CAD build for the part. Positions are in the model's coordinates, mm. Face numbers are marked on the shaded views. A direction names the side the tool comes from. Round coordinates to 2 decimals unless told otherwise and drop trailing zeros. Loops run counter-clockwise (first coordinate to the right, second up) from the corner with the lowest first, then second, coordinate; pieces in that order, holes last.
```python
from build123d import *

# Parameters (mm, degrees)
F3_D = 12
F4_R = 2
F5_R = 4


with BuildPart() as f1:
    # F0 (on Front) → F1 (revolve)
    with BuildSketch(Plane.XZ):
        Polygon((22, 17), (17.25, 17), (17.25, 0), (47.5, 0), (47.5, 10), (22, 10), align=None)
    revolve(axis=Axis((0, 0, 4.398516), (0, 0, -1)))

    # F3 (through all)
    with Locations(Plane.XY.offset(10)):
        with Locations((-26.516504, 26.516504), (-26.516504, -26.516504), (26.516504, -26.516504), (26.516504, 26.516504)):
            Hole(F3_D / 2)

    # F4
    f4_edges = [f1.edges().sort_by_distance(p)[0] for p in [
        (-22, 0, 17),
        (-47.5, 0, 10),
    ]]
    fillet(f4_edges, radius=F4_R)

    # F5
    f5_edges = [f1.edges().sort_by_distance(p)[0] for p in [
        (-22, 0, 10),
    ]]
    fillet(f5_edges, radius=F5_R)


solid = f1.part
```
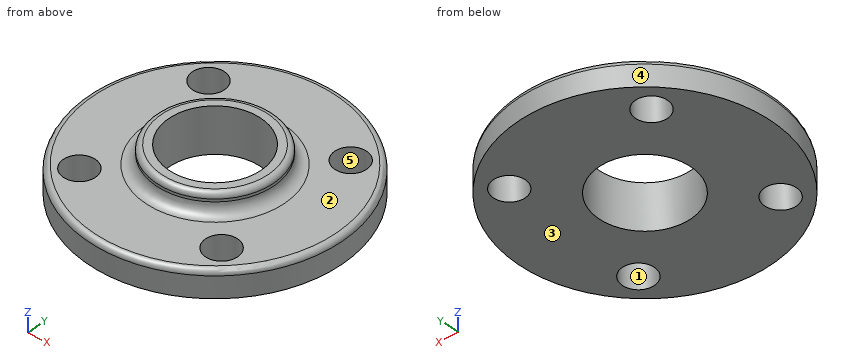
Item 1: Flat gauge pins, fed straight in: P1, Ø11, axis at x = -26.52, y = -26.52, coming from the -Z side; P2, Ø3, axis at x = -21.5, z = 7, coming from the -Y side; P3, Ø5, axis at x = 19.5, z = 6.5, coming from the -Y side; P4, Ø2, axis at x = 21, y = 5, coming from the +Z side. Where does each tip first touch, or does it go through?
Answers follow:
P1: passes through
P2: stops at y = -43.08
P3: stops at y = -44.35
P4: stops at z = 16.91
Item 2: Cut at D-D, the plane x = 31. State how many separate pieces and enclosed holes the cut face has, plus the area to 3 significant figures.
Answers follow:
separate pieces: 3
enclosed holes: 0
area: 558 mm2
Item 3: 3-axis set-ups, long thin cutter, end or side, ignore diameter. For the marked faces 1 and 2: which of +Z, -Z, +X, -X, +Y, -Y reach the whole face in a straight line?
Answers follow:
face 1: +Z, -Z
face 2: +Z
Item 4: Two-plate mould, pull along Y, no slides. Class the marked faces 3, 4 and 5: released by +Y, released by -Y, zero draft, split by the parting line, or undercut.
Answers follow:
face 3: zero draft
face 4: split by the parting line
face 5: undercut
Item 5: Cut at C-C, the plane z = 2.5. Give the cut face in (x, y), plus the area to 3 significant figures.
Answers follow:
outline: circle Ø95 at (0, 0); hole circle Ø12 at (-26.52, -26.52); hole circle Ø12 at (-26.52, 26.52); hole circle Ø34.5 at (0, 0); hole circle Ø12 at (26.52, -26.52); hole circle Ø12 at (26.52, 26.52)
area: 5,700 mm2
Item 6: Cut at A-A, the plane x = 0. Give the cut face in (y, z).
Answers follow:
outline: (-47.5, 0) - (-17.25, 0) - (-17.25, 17) - (-20, 17) arc R2 ccw to (-22, 15) - (-22, 14) arc R4 cw to (-26, 10) - (-45.5, 10) arc R2 ccw to (-47.5, 8) - close; (17.25, 0) - (47.5, 0) - (47.5, 8) arc R2 ccw to (45.5, 10) - (26, 10) arc R4 cw to (22, 14) - (22, 15) arc R2 ccw to (20, 17) - (17.25, 17) - close
Item 7: Probe line 1 (X direction, y = 0, z = 8); line 2 (X direction, y = 28.5, z = 2.25); line 3 (Y direction, x = -29, z = 7.5). List the from-to ranges inside material, lowest first.
Answers follow:
line 1: x = -47.5 to -17.25, 17.25 to 47.5
line 2: x = -38 to -32.18, -20.85 to 20.85, 32.18 to 38
line 3: y = -37.62 to -31.98, -21.05 to 21.05, 31.98 to 37.62
